Can you work these out from the model? Positions are in its coordinate system, mm. A direction names the side the tool comes from. Give positions to 0.01 mm unless a question says otherwise; leave off trailing zeros. Write each loop counter-clockwise with the first axis right and the second up, starting at its lowest first coordinate (ties: lowest second). Pieces come first, ordered by that corner, then holes.
```python
from build123d import *

# Parameters (mm, degrees)
F0_R     = 6.35
F1_DEPTH = 6.35
F2_DEPTH = 7.62


with BuildPart() as f1:
    # F0 (on Top) → F1 (new body)
    with BuildSketch(Plane.XY):
        Polygon((34.710955, 45.041551), (9.310955, 45.041551), (9.310955, 32.341551), (9.310955, 6.941551), (9.310955, -18.458449), (9.310955, -43.858449), (9.310955, -56.558449), (34.710955, -56.558449), align=None)
        with Locations((22.010955, -43.858449)):
            Circle(F0_R, mode=Mode.SUBTRACT)
        with Locations((22.010955, -18.458449)):
            Circle(F0_R, mode=Mode.SUBTRACT)
        with Locations((22.010955, 6.941551)):
            Circle(F0_R, mode=Mode.SUBTRACT)
        with Locations((22.010955, 32.341551)):
            Circle(F0_R, mode=Mode.SUBTRACT)
    extrude(amount=F1_DEPTH)

    # F0 (on Top) → F2 (join)
    with BuildSketch(Plane.XY):
        with Locations((22.010955, -18.458449)):
            Circle(F0_R)
        with Locations((22.010955, -43.858449)):
            Circle(F0_R)
        with Locations((22.010955, 6.941551)):
            Circle(F0_R)
        with Locations((22.010955, 32.341551)):
            Circle(F0_R)
    extrude(amount=F2_DEPTH)


solid = f1.part
```
1) Suppose I cut it at D-D on x = 21.75. Write out the boundary of the cut face in (y, z), plus the area to 3 significant figures.
Values follow:
outline: (-56.56, 0) - (45.04, 0) - (45.04, 6.35) - (38.69, 6.35) - (38.69, 7.62) - (26, 7.62) - (26, 6.35) - (13.29, 6.35) - (13.29, 7.62) - (0.6, 7.62) - (0.6, 6.35) - (-12.11, 6.35) - (-12.11, 7.62) - (-24.8, 7.62) - (-24.8, 6.35) - (-37.51, 6.35) - (-37.51, 7.62) - (-50.2, 7.62) - (-50.2, 6.35) - (-56.56, 6.35) - close
area: 710 mm2
2) Suppose I cut it at C-C on y = 27. Write out the boundary of the cut face in (x, z), plus the area to 3 significant figures.
Values follow:
outline: (9.31, 0) - (34.71, 0) - (34.71, 6.35) - (25.44, 6.35) - (25.44, 7.62) - (18.58, 7.62) - (18.58, 6.35) - (9.31, 6.35) - close
area: 170 mm2
3) Suppose I cut it at A-A on y = 6. Write out the boundary of the cut face in (x, z), plus the area to 3 significant figures.
Values follow:
outline: (9.31, 0) - (34.71, 0) - (34.71, 6.35) - (28.29, 6.35) - (28.29, 7.62) - (15.73, 7.62) - (15.73, 6.35) - (9.31, 6.35) - close
area: 177 mm2
4) Please list where these lines run through material, in increasing order: L1, parallel to Y at x = 25.5, z = 7.25; L2, parallel to Z at x = 30.5, y = -14.5; L3, parallel to X at y = 34.5, z = 6.5.
Values follow:
L1: y = -49.16 to -38.55, -23.76 to -13.15, 1.64 to 12.25, 27.04 to 37.65
L2: z = 0 to 6.35
L3: x = 16.04 to 27.98
5) If we mould it in two halves opening along Y, with no side actions, what happens to faces 1 (the face through (22, -5, 6.35)), 2 (the face through (22, -5, 0)), 3 (the face through (22, -56.558, 3))? For each: +Y half, -Y half, draft (parallel to the pull), parting line (faces both ways), or undercut.
Values follow:
face 1: undercut
face 2: draft
face 3: -Y half
6) For faces 4 (the face through (28.068, 34.249, 6.976)), 5 (the face through (22, -18, 7.62)), which set-ups out of +Z, -Z, +X, -X, +Y, -Y let a thin tool reach every point of the face, with its end or its side?
Values follow:
face 4: +Z
face 5: +Z, +X, -X, +Y, -Y
7) Suppose I cut it at B-B on x = 27.5. Write out the boundary of the cut face in (y, z).
Values follow:
outline: (-56.56, 0) - (45.04, 0) - (45.04, 6.35) - (35.53, 6.35) - (35.53, 7.62) - (29.15, 7.62) - (29.15, 6.35) - (10.13, 6.35) - (10.13, 7.62) - (3.75, 7.62) - (3.75, 6.35) - (-15.27, 6.35) - (-15.27, 7.62) - (-21.65, 7.62) - (-21.65, 6.35) - (-40.67, 6.35) - (-40.67, 7.62) - (-47.05, 7.62) - (-47.05, 6.35) - (-56.56, 6.35) - close
